from build123d import *

# Parameters (mm, degrees)
SKETCH1_R           = 1.5
SKETCH1_R_2         = 4.925
SKETCH1_W           = 5.35
SKETCH1_H           = 30.5
SKETCH1_W_2         = 6.4
SKETCH1_H_2         = 9.4
BOSS_EXTRUDE1_DEPTH = 6.4
SKETCH2_R           = 1.5
SKETCH2_W           = 6.4
SKETCH2_H           = 9.9
SKETCH2_W_2         = 9.9
SKETCH2_H_2         = 6.4
SKETCH2_H_3         = 9.8
CUT_EXTRUDE1_DEPTH  = 415.760486883


with BuildPart() as part:
    # Sketch1 → Boss-Extrude1 (new body)
    with BuildSketch(Plane(origin=(0, 0, 0), x_dir=(0, 0, -1), z_dir=(1, 0, 0))):
        Polygon((-37.634998875, 41.275232149), (210.165001125, 41.275232149), (246.265001125, 5.175232149), (246.265001125, -333.674767851), (190.325001125, -333.674767851), (175.325001125, -318.674767851), (-18.721689147, -318.674767851), (-33.721689147, -333.674767851), (-73.734998875, -333.674767851), (-73.734998875, 5.175232149), align=None)
        with Locations((6.165001125, 34.475232149)):
            Circle(SKETCH1_R, mode=Mode.SUBTRACT)
        with Locations((86.365001125, 34.475232149)):
            Circle(SKETCH1_R, mode=Mode.SUBTRACT)
        with Locations((166.365001125, 34.475232149)):
            Circle(SKETCH1_R, mode=Mode.SUBTRACT)
        with Locations((86.365001125, -259.124767851)):
            Circle(SKETCH1_R, mode=Mode.SUBTRACT)
        with Locations((166.465001125, -259.124767851)):
            Circle(SKETCH1_R, mode=Mode.SUBTRACT)
        with Locations((6.265001125, -259.124767851)):
            Circle(SKETCH1_R, mode=Mode.SUBTRACT)
        with Locations((239.465001125, -29.824767851)):
            Circle(SKETCH1_R, mode=Mode.SUBTRACT)
        with Locations((239.465001125, -136.224767851)):
            Circle(SKETCH1_R, mode=Mode.SUBTRACT)
        with Locations((239.465001125, -242.624767851)):
            Circle(SKETCH1_R, mode=Mode.SUBTRACT)
        with Locations((-66.934998875, -242.624767851)):
            Circle(SKETCH1_R, mode=Mode.SUBTRACT)
        with Locations((-66.934998875, -136.224767851)):
            Circle(SKETCH1_R, mode=Mode.SUBTRACT)
        with Locations((-66.934998875, -29.824767851)):
            Circle(SKETCH1_R, mode=Mode.SUBTRACT)
        with Locations((224.265001125, 13.800232149)):
            Circle(SKETCH1_R_2, mode=Mode.SUBTRACT)
        with Locations((-51.734998875, 13.800232149)):
            Circle(SKETCH1_R_2, mode=Mode.SUBTRACT)
        with Locations((228.265001125, -300.824767851)):
            Circle(SKETCH1_R, mode=Mode.SUBTRACT)
        with Locations((196.265001125, -300.824767851)):
            Circle(SKETCH1_R, mode=Mode.SUBTRACT)
        Polygon((-34.371689147, -25.324767851), (-34.371689147, -206.824767851), (189.675001125, -206.824767851), (189.675001125, -25.324767851), (157.825001125, 6.525232149), (-2.521689147, 6.525232149), align=None, mode=Mode.SUBTRACT)
        with Locations((-59.409998875, -228.624767851)):
            Rectangle(SKETCH1_W, SKETCH1_H, mode=Mode.SUBTRACT)
        Polygon((230.451321469, -30.923586412), (229.208680782, -30.923586412), (228.330001125, -31.802266068), (228.330001125, -40.046830544), (229.208680782, -40.925510201), (230.451321469, -40.925510201), (231.330001125, -40.046830544), (231.330001125, -31.802266068), align=None, mode=Mode.SUBTRACT)
        Polygon((215.878301984, -58.680508661), (212.771700266, -58.680508661), (210.575001125, -56.483809519), (210.575001125, -46.377207802), (212.771700266, -44.180508661), (215.878301984, -44.180508661), (218.075001125, -46.377207802), (218.075001125, -56.483809519), align=None, mode=Mode.SUBTRACT)
        Polygon((200.330001125, -31.802266068), (199.451321469, -30.923586412), (198.208680782, -30.923586412), (197.330001125, -31.802266068), (197.330001125, -40.046830544), (198.208680782, -40.925510201), (199.451321469, -40.925510201), (200.330001125, -40.046830544), align=None, mode=Mode.SUBTRACT)
        Polygon((230.451321469, -61.923586412), (229.208680782, -61.923586412), (228.330001125, -62.802266068), (228.330001125, -71.046830544), (229.208680782, -71.925510201), (230.451321469, -71.925510201), (231.330001125, -71.046830544), (231.330001125, -62.802266068), align=None, mode=Mode.SUBTRACT)
        Polygon((199.451321469, -61.923586412), (198.208680782, -61.923586412), (197.330001125, -62.802266068), (197.330001125, -71.046830544), (198.208680782, -71.925510201), (199.451321469, -71.925510201), (200.330001125, -71.046830544), (200.330001125, -62.802266068), align=None, mode=Mode.SUBTRACT)
        with Locations((239.465001125, -44.824767851)):
            Rectangle(SKETCH1_W_2, SKETCH1_H_2, mode=Mode.SUBTRACT)
    extrude(amount=BOSS_EXTRUDE1_DEPTH)

    # Sketch2 → Cut-Extrude1 (cut, through all)
    with BuildSketch(Plane(origin=(6.4, 0, 0), x_dir=(0, 0, -1), z_dir=(1, 0, 0))):
        with Locations((22.965001125, -275.874767851)):
            Circle(SKETCH2_R)
        with Locations((86.365001125, -311.024767851)):
            Circle(SKETCH2_R)
        with Locations((239.465001125, -257.624767851)):
            Rectangle(SKETCH2_W, SKETCH2_H)
        with Locations((239.465001125, -227.624767851)):
            Rectangle(SKETCH2_W, SKETCH2_H)
        with Locations((-66.934998875, -257.624767851)):
            Rectangle(SKETCH2_W, SKETCH2_H)
        with Locations((-66.934998875, -227.624767851)):
            Rectangle(SKETCH2_W, SKETCH2_H)
        with Locations((-66.934998875, -151.224767851)):
            Rectangle(SKETCH2_W, SKETCH2_H)
        with Locations((-66.934998875, -121.224767851)):
            Rectangle(SKETCH2_W, SKETCH2_H)
        with Locations((-66.934998875, -44.824767851)):
            Rectangle(SKETCH2_W, SKETCH2_H)
        with Locations((-66.934998875, -14.824767851)):
            Rectangle(SKETCH2_W, SKETCH2_H)
        with Locations((239.465001125, -121.224767851)):
            Rectangle(SKETCH2_W, SKETCH2_H)
        with Locations((239.465001125, -151.224767851)):
            Rectangle(SKETCH2_W, SKETCH2_H)
        with Locations((239.465001125, -14.824767851)):
            Rectangle(SKETCH2_W, SKETCH2_H)
        with Locations((239.465001125, -44.824767851)):
            Rectangle(SKETCH2_W, SKETCH2_H)
        with Locations((71.365001125, -259.124767851)):
            Rectangle(SKETCH2_W_2, SKETCH2_H_2)
        with Locations((101.365001125, -259.124767851)):
            Rectangle(SKETCH2_W_2, SKETCH2_H_2)
        with Locations((151.465001125, -259.124767851)):
            Rectangle(SKETCH2_W_2, SKETCH2_H_2)
        with Locations((181.465001125, -259.124767851)):
            Rectangle(SKETCH2_W_2, SKETCH2_H_2)
        with Locations((151.365001125, 34.475232149)):
            Rectangle(SKETCH2_W_2, SKETCH2_H_2)
        with Locations((181.365001125, 34.475232149)):
            Rectangle(SKETCH2_W_2, SKETCH2_H_2)
        with Locations((-8.734998875, -259.124767851)):
            Rectangle(SKETCH2_W_2, SKETCH2_H_2)
        with Locations((21.265001125, -259.124767851)):
            Rectangle(SKETCH2_W_2, SKETCH2_H_2)
        with Locations((71.365001125, 34.475232149)):
            Rectangle(SKETCH2_W_2, SKETCH2_H_2)
        with Locations((101.365001125, 34.475232149)):
            Rectangle(SKETCH2_W_2, SKETCH2_H_2)
        with Locations((-8.834998875, 34.475232149)):
            Rectangle(SKETCH2_W_2, SKETCH2_H_2)
        with Locations((21.165001125, 34.475232149)):
            Rectangle(SKETCH2_W_2, SKETCH2_H_2)
        with Locations((22.965001125, -294.324767851)):
            Rectangle(SKETCH2_W, SKETCH2_H_3)
    extrude(amount=-CUT_EXTRUDE1_DEPTH, mode=Mode.SUBTRACT)


solid = part.part
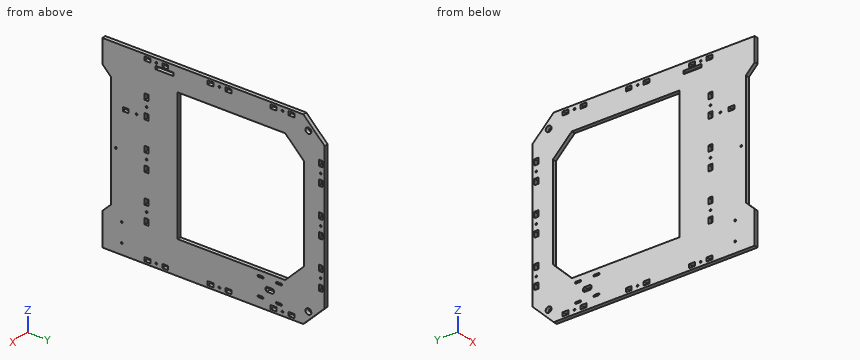
Model file for the job. Use its own axes, mm. Give positions to 0.01 mm unless a question says otherwise; leave off trailing zeros. Order: outer loops, then holes, each group sorted by start corner. A loop starts at its lowest first (then second) coordinate and runs counter-clockwise, first axis right, second up. Notation, with made-up numbers: (54.25, -6.5) -> (86.25, -6.5) arc R15 ccw to (86.25, 1.5) -> close; hole circle Ø9 at (87.25, 10). An arc over 180 degrees is marked (long way). Use CSV: the item, a comma, the result in double quotes.
1. Drill centre lines: line 1 along Y through (x, z) = (3, -25.5); line 2 along Z through (x, y) = (1.5, -63) (3 decimals); line 3 along Y through (x, z) = (5.75, -98). Where is each one in solid material? Low to high. Write a range as from..to.
Outcome:
line 1,"-318.67..-299.22, -289.42..-262.32, -255.92..-206.82, 6.53..31.28, 37.68..41.28"
line 2,"-246.265..-231.33, -228.33..-200.33, -197.33..-189.675, 34.372..73.735"
line 3,"-318.67..-262.32, -255.92..-206.82, 6.53..31.28, 37.68..41.28"
2. Band-saw the part on B-B, the plane y = -188.5. Give the cut face in (x, z) (3 decimals), then the cut area to 3 significant figures.
Outcome:
outline,"(0, -246.265) -> (6.4, -246.265) -> (6.4, -189.675) -> (0, -189.675) -> close; (0, 34.372) -> (6.4, 34.372) -> (6.4, 73.735) -> (0, 73.735) -> close"
area,"614 mm²"
3. Band-saw the part on A-A, the plane z = -44. Give the cut face in (x, y), then the cut area to 3 significant figures.
Outcome:
outline,"(0, -318.67) -> (6.4, -318.67) -> (6.4, -206.82) -> (0, -206.82) -> close; (0, 6.53) -> (6.4, 6.53) -> (6.4, 41.28) -> (0, 41.28) -> close"
area,"938 mm²"
4. Band-saw the part on C-C, the plane x = 4.5. Count the separate pieces of the cut face and the enclosed holes in it, then the cut area to 3 significant figures.
Outcome:
separate pieces,"1"
enclosed holes,"50"
area,"66,500 mm²"
